Check sheet for the modelled part. Datum: model origin and axes. Units: mm. Face numbers are marked on the shaded views. Round coordinates to 2 decimals unless told otherwise and drop trailing zeros. Answer in a Markdown table with one row per item. Add a question column.
1. Material ranges on L1, parallel to Y at x = 127.5, z = -26; L2, parallel to Z at x = 34.5, y = 83; L3, parallel to X at y = 49, z = 383, recorded low to high. Write a range as from..to.
2. Depth check by flat-ended pin: P1, Ø4, axis at x = 124, y = 64.5, coming from the -Z side. Enter the tip coordinate at first touch or a pass-through.
3. Draft check along Z on the marked faces 1 and 2. Enter one of: +Z half, -Z half, draft (parallel to the pull), parting line (faces both ways), or undercut.
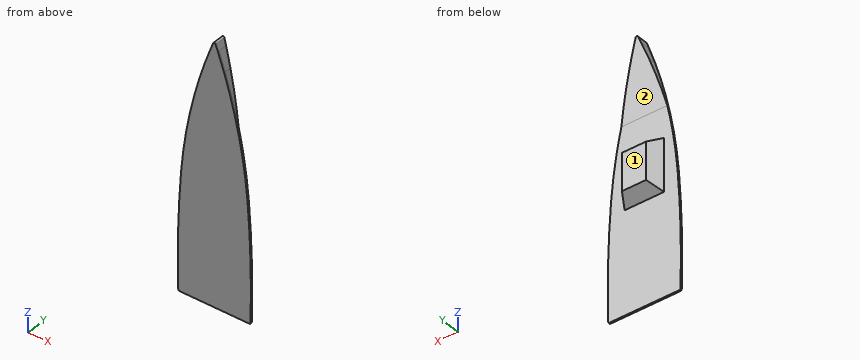
```python
from build123d import *

# Parameters (mm, degrees)
BOSS_EXTRUDE1_DEPTH     = 12.7
SKETCH2_W               = 304.8
SKETCH2_H               = 406.4
BOSS_EXTRUDE2_DEPTH     = 101.6
BOSS_EXTRUDE2_TAPER     = 30
BOSS_EXTRUDE3_DEPTH     = 74.997994
SKETCH7_W               = 508
SKETCH7_H               = 565.262345734
CUT_EXTRUDE_THIN1_DEPTH = 88.9


with BuildPart() as part:
    # Sketch1 → Boss-Extrude1 (new body)
    with BuildSketch(Plane(origin=(0, 0, 0), x_dir=(1, 0, 0), z_dir=(0, 1, 0))):
        with BuildLine():
            Line((282.178632733, 648.295571298), (-266.742186919, 648.295571298))
            add(Edge.make_bspline(
                [(-266.742186919, 648.295571298), (-267.071605745, 648.295571298), (-267.395635709, 648.263919559), (-267.873929001, 648.170912239), (-268.032058898, 648.132267139), (-268.345661652, 648.039370684), (-268.50177233, 647.984795184), (-268.956632468, 647.800648785), (-269.244615581, 647.650355056), (-269.790494311, 647.295478174), (-270.050162442, 647.088526762), (-270.517954254, 646.635397593), (-270.728625138, 646.388172726), (-271.009326112, 645.985928841), (-271.097290935, 645.845887253), (-271.257701503, 645.560682787), (-271.330552726, 645.415064516), (-271.527511364, 644.969353179), (-271.630228502, 644.660487559), (-271.776102581, 644.018329571), (-271.817451265, 643.692751749), (-271.827054921, 643.363460144)],
                knots=[0, 0, 0, 0, 0.125, 0.125, 0.1875, 0.1875, 0.25, 0.25, 0.375, 0.375, 0.5, 0.5, 0.625, 0.625, 0.6875, 0.6875, 0.75, 0.75, 0.875, 0.875, 1, 1, 1, 1], degree=3))
            add(Edge.make_bspline(
                [(-271.827054921, 643.363460144), (-275.619083406, 513.341805118), (-276.544805746, 362.627319415), (-273.085954654, 195.044872043), (-271.031571931, 119.847777975), (-268.671598158, 56.063015866), (-263.132069886, -66.069662637), (-257.433335824, -160.037587725), (-250.764013725, -248.746196584), (-248.487290338, -276.985560905), (-240.18277645, -371.092813978), (-227.549965864, -472.778666072), (-212.610504693, -566.462025361), (-203.222738687, -622.637020096), (-193.844144823, -673.237560968), (-182.290724358, -729.93756534), (-174.271233518, -767.830757671), (-162.896711093, -818.371776774), (-149.252675491, -874.959703685), (-120.211836445, -987.796815407), (-92.347727316, -1081.139961257), (-67.767522398, -1155.104428702)],
                knots=[0.00273139, 0.00273139, 0.00273139, 0.00273139, 0.21875, 0.253283969, 0.28125, 0.34375, 0.359375, 0.484375, 0.5, 0.506595501, 0.53125, 0.65625, 0.67558323, 0.6875, 0.75, 0.760136029, 0.78125, 0.8125, 0.84375, 0.875, 1, 1, 1, 1], degree=3))
            add(Edge.make_bspline(
                [(-67.767522398, -1155.104428702), (-52.556679091, -1200.875484247), (-36.785485559, -1245.497662336), (-19.856460022, -1290.661446214)],
                knots=[0, 0, 0, 0, 1, 1, 1, 1], degree=3))
            ThreePointArc((-19.856460022, -1290.661446214), (-10.585699255, -1315.137822671), (-1.146808464, -1339.549855571))
            add(Edge.make_bspline(
                [(-1.146808464, -1339.549855571), (-0.800991585, -1340.435186307), (0.157660597, -1342.101440742), (2.269639684, -1344.064855704), (4.866902728, -1345.317723875), (6.767749431, -1345.604428702), (7.718222907, -1345.604428702)],
                knots=[0.808269867, 0.808269867, 0.808269867, 0.808269867, 0.8562024, 0.904134933, 0.952067467, 0.99999997, 0.99999997, 0.99999997, 0.99999997], degree=3))
            add(Edge.make_bspline(
                [(16.583254278, -1339.549855571), (16.237437398, -1340.435186307), (15.278785216, -1342.101440742), (13.16680613, -1344.064855704), (10.569543086, -1345.317723875), (8.668696382, -1345.604428702), (7.718222907, -1345.604428702)],
                knots=[0.808269867, 0.808269867, 0.808269867, 0.808269867, 0.8562024, 0.904134933, 0.952067467, 1, 1, 1, 1], degree=3))
            ThreePointArc((16.583254278, -1339.549855571), (26.022145069, -1315.137822671), (35.292905835, -1290.661446214))
            add(Edge.make_bspline(
                [(83.203968212, -1155.104428702), (67.993124905, -1200.875484247), (52.221931373, -1245.497662336), (35.292905835, -1290.661446214)],
                knots=[0, 0, 0, 0, 1, 1, 1, 1], degree=3))
            add(Edge.make_bspline(
                [(287.263500734, 643.363460144), (291.055529219, 513.341805118), (291.98125156, 362.627319415), (288.522400468, 195.044872043), (286.468017744, 119.847777975), (284.108043971, 56.063015866), (278.568515699, -66.069662637), (272.869781637, -160.037587725), (266.200459538, -248.746196584), (263.923736151, -276.985560905), (255.619222264, -371.092813978), (242.986411678, -472.778666072), (228.046950506, -566.462025361), (218.659184501, -622.637020096), (209.280590637, -673.237560968), (197.727170171, -729.93756534), (189.707679331, -767.830757671), (178.333156907, -818.371776774), (164.689121304, -874.959703685), (135.648282259, -987.796815407), (107.78417313, -1081.139961257), (83.203968212, -1155.104428702)],
                knots=[0.00273139, 0.00273139, 0.00273139, 0.00273139, 0.21875, 0.253283969, 0.28125, 0.34375, 0.359375, 0.484375, 0.5, 0.506595501, 0.53125, 0.65625, 0.67558323, 0.6875, 0.75, 0.760136029, 0.78125, 0.8125, 0.84375, 0.875, 1, 1, 1, 1], degree=3))
            add(Edge.make_bspline(
                [(287.263500734, 643.363460144), (287.253897353, 643.692742337), (287.212682478, 644.015685877), (287.105404307, 644.490986496), (287.062014477, 644.64789), (286.959654545, 644.958572893), (286.900349557, 645.112951735), (286.70240916, 645.561902127), (286.54331042, 645.845111412), (286.171615525, 646.379810232), (285.956670805, 646.632890984), (285.489257001, 647.086264872), (285.235568792, 647.289160564), (284.824662826, 647.557338937), (284.681966904, 647.640918903), (284.392063507, 647.792397056), (284.244309066, 647.860727323), (283.491814956, 648.166105966), (282.837451466, 648.295571298), (282.178632733, 648.295571298)],
                knots=[0, 0, 0, 0, 0.125, 0.125, 0.1875, 0.1875, 0.25, 0.25, 0.375, 0.375, 0.5, 0.5, 0.625, 0.625, 0.6875, 0.6875, 0.75, 0.75, 1, 1, 1, 1], degree=3))
        make_face()
    extrude(amount=BOSS_EXTRUDE1_DEPTH)

    # Sketch2 → Boss-Extrude2 (add)
    with BuildSketch(Plane(origin=(0, 12.7, 0), x_dir=(1, 0, 0), z_dir=(0, 1, 0))):
        with Locations((7.718222907, -348.654428702)):
            Rectangle(SKETCH2_W, SKETCH2_H)
    extrude(amount=BOSS_EXTRUDE2_DEPTH, taper=BOSS_EXTRUDE2_TAPER)

    # Sketch4 → Boss-Extrude3 (add)
    with BuildSketch(Plane(origin=(0, 12.7, 0), x_dir=(1, 0, 0), z_dir=(0, 1, 0))):
        with BuildLine():
            Line((-170.289770142, -785.339473227), (185.726215956, -785.339473227))
            add(Edge.make_bspline(
                [(83.203968212, -1155.104428702), (107.78417313, -1081.139961257), (135.648282259, -987.796815407), (164.689121304, -874.959703685), (176.435611281, -826.241748411), (183.262218235, -796.353082345), (185.726215956, -785.339473227)],
                knots=[0.00273139, 0.00273139, 0.00273139, 0.00273139, 0.12773139, 0.15898139, 0.19023139, 0.208443099, 0.208443099, 0.208443099, 0.208443099], degree=3))
            add(Edge.make_bspline(
                [(35.292905835, -1290.661446214), (52.221931373, -1245.497662336), (67.993124905, -1200.875484247), (83.203968212, -1155.104428702)],
                knots=[0, 0, 0, 0, 1, 1, 1, 1], degree=3))
            ThreePointArc((35.292905835, -1290.661446214), (26.022145069, -1315.137822671), (16.583254278, -1339.549855571))
            add(Edge.make_bspline(
                [(7.718222907, -1345.604428702), (8.668696382, -1345.604428702), (10.569543086, -1345.317723875), (13.16680613, -1344.064855704), (15.278785216, -1342.101440742), (16.237437398, -1340.435186307), (16.583254278, -1339.549855571)],
                knots=[0.808269867, 0.808269867, 0.808269867, 0.808269867, 0.8562024, 0.904134933, 0.952067467, 1, 1, 1, 1], degree=3))
            add(Edge.make_bspline(
                [(-1.146808464, -1339.549855571), (-0.800991585, -1340.435186307), (0.157660597, -1342.101440742), (2.269639684, -1344.064855704), (4.866902728, -1345.317723875), (6.767749431, -1345.604428702), (7.718222907, -1345.604428702)],
                knots=[0.808269867, 0.808269867, 0.808269867, 0.808269867, 0.8562024, 0.904134933, 0.952067467, 0.99999997, 0.99999997, 0.99999997, 0.99999997], degree=3))
            ThreePointArc((-1.146808464, -1339.549855571), (-10.585699255, -1315.137822671), (-19.856460022, -1290.661446214))
            add(Edge.make_bspline(
                [(-67.767522398, -1155.104428702), (-52.556679091, -1200.875484247), (-36.785485559, -1245.497662336), (-19.856460022, -1290.661446214)],
                knots=[0, 0, 0, 0, 1, 1, 1, 1], degree=3))
            add(Edge.make_bspline(
                [(-170.289770142, -785.339473227), (-167.825772422, -796.353082345), (-160.999165467, -826.241748411), (-149.252675491, -874.959703685), (-120.211836445, -987.796815407), (-92.347727316, -1081.139961257), (-67.767522398, -1155.104428702)],
                knots=[0.794288291, 0.794288291, 0.794288291, 0.794288291, 0.8125, 0.84375, 0.875, 1, 1, 1, 1], degree=3))
        make_face()
    extrude(amount=BOSS_EXTRUDE3_DEPTH)

    # Sketch7 → Cut-Extrude-Thin1 (cut)
    with BuildSketch(Plane(origin=(0, -90.799805475, 12.154612278), x_dir=(1, 0, 0), z_dir=(0, 0.991159167, -0.132678207))):
        with Locations((7.718222907, -1062.71260383)):
            Rectangle(SKETCH7_W, SKETCH7_H)
    extrude(amount=CUT_EXTRUDE_THIN1_DEPTH, mode=Mode.SUBTRACT)


solid = part.part
```
Answer key:
| question | item | result |
|---|---|---|
| 1 | L1 | y = 0..12.7 |
| 1 | L2 | z = 186.04..511.27 |
| 1 | L3 | x = -123.72..139.16 |
| 2 | P1 | stops at z = 174.21 |
| 3 | face 1 | draft |
| 3 | face 2 | undercut |
